Design review of the part shown in the three views and the two pictorial views. Dimensions are in mm from the part's minimum x, y and z. A direction names the side the tool comes from. Give positions to 0.01 mm unless a question says otherwise; leave off trailing zeros. Write each loop counter-clockwise with the first axis right and the second up, starting at its lowest first coordinate (ties: lowest second). Pieces come first, ordered by that corner, then holes. Notation, with made-up numbers: (-23.5, 41.25) -> (28.5, 41.25) arc R20 cw to (28.5, 71.25) -> close; hole circle Ø3 at (69.5, 37). An arc over 180 degrees is marked (long way). Return JSON: item names as keys, results as strings. Group by question number.
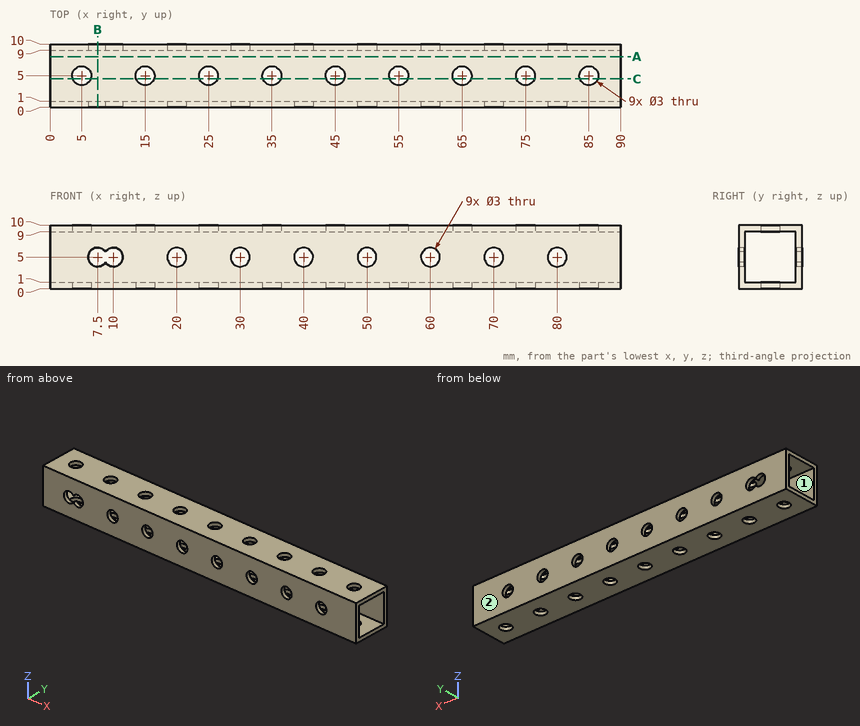
Q1. Take a section at A-A, the plane y = 8. Give the boundary of the cut face in (x, z), plus the area to 3 significant figures.
Q2. Insertion check: pin 1 (2 mm diameter, centred on x = 68, y = 7.5, fed in from -Z); pin 2 (1.8 mm diameter, centred on x = 10, z = 5, fed in from -Y). Each pin has a flat end and moves straight along its axis. Give the tip position at first contact, or say it passes through.
Q3. Take a section at B-B, the plane x = 7.5. Give the boundary of the cut face in (y, z).
Q4. Take a section at C-C, the plane y = 4.5. Count the separate pieces of the cut face and the enclosed holes in it, plus the area to 3 significant figures.
Q5. Tool access review of the marked faces 1 and 2: name each direction out of +Z, -Z, +X, -X, +Y, -Y from which nothing blocks a thin tool from reaching the whole face with its end or side.
Q6. For L1, parallel to Y at x = 75, z = 4.25; L2, parallel to Y at x = 5, z = 9.65, list the stretches that pass through material, from the lowest coordinate up. Write a range as from..to.
Final values:
{
 "1": {"outline": "(0, 0) -> (90, 0) -> (90, 1) -> (0, 1) -> close; (0, 9) -> (90, 9) -> (90, 10) -> (0, 10) -> close", "area": "180 mm²"},
 "2": {"pin 1": "stops at z = 0", "pin 2": "passes through"},
 "3": {"outline": "(0, 0) -> (10, 0) -> (10, 3.5) -> (9, 3.5) -> (9, 1) -> (1, 1) -> (1, 3.5) -> (0, 3.5) -> close; (0, 6.5) -> (1, 6.5) -> (1, 9) -> (9, 9) -> (9, 6.5) -> (10, 6.5) -> (10, 10) -> (0, 10) -> close"},
 "4": {"separate pieces": "20", "enclosed holes": "0", "area": "129 mm²"},
 "5": {"face 1": "+X, -X", "face 2": "+Z, -Z, +X, -X, +Y"},
 "6": {"L1": "y = 0..1, 9..10", "L2": "y = 0..3.5, 6.5..10"}
}
